Design review of the part built by this model. Coordinates are the model's own, in mm. A direction names the side the tool comes from. Give positions to 0.01 mm unless a question says otherwise; leave off trailing zeros. Loops run counter-clockwise (first coordinate to the right, second up) from the corner with the lowest first, then second, coordinate; pieces in that order, holes last. Notation, with made-up numbers: (14, 81.25) - (65, 81.25) arc R11 cw to (65, 86.25) - close; hole circle Ø6 at (42, 63). An arc over 180 degrees is marked (long way). Write each question's results on one line, items separated by ' | '.
Autodesk Inventor part; units mm, degrees
ref_plane "YZ Plane" through (0, 0, 0) normal (1, 0, 0) x (0, 1, 0)
ref_plane "XZ Plane" through (0, 0, 0) normal (0, 1, 0) x (-1, 0, 0)
ref_plane "XY Plane" through (0, 0, 0) normal (0, 0, 1) x (1, 0, 0)
sketch "Sketch1" plane through (0, 0, 0) normal (0, 1, 0) x (-1, 0, 0)
  circle A0 centre (0, 0) radius 10
  dimension "d0" = 20
extrude "Extrusion1" add sketch "Sketch1" along normal blind 2
sketch "Sketch2" plane through (0, 2, 0) normal (0, 1, 0) x (1, 0, 0)
  circle A0 centre (0, 0) radius 5.875
  dimension "d3" = 11.75
extrude "Extrusion2" cut sketch "Sketch2" against normal blind 1
sketch "Sketch3" plane through (0, 1, 0) normal (0, 1, 0) x (1, 0, 0)
  circle A0 centre (0, 0) radius 2
  dimension "d6" = 4
extrude "Extrusion3" cut sketch "Sketch3" against normal through all
properties part number "M3Bearing_Holder"
Item 1: We need section B-B on z = 0. Give the boundary of the cut face in (x, y) (3 decimals), then the cut area to 4 significant figures.
Output values:
outline: (-10, 0) - (-2, 0) - (-2, 1) - (-5.875, 1) - (-5.875, 2) - (-10, 2) - close; (2, 0) - (10, 0) - (10, 2) - (5.875, 2) - (5.875, 1) - (2, 1) - close | area: 24.25 mm²
Item 2: We need section D-D on x = 3. Give the boundary of the cut face in (y, z).
Output values:
outline: (0, -9.54) - (2, -9.54) - (2, -5.05) - (1, -5.05) - (1, 5.05) - (2, 5.05) - (2, 9.54) - (0, 9.54) - close
Item 3: Clearance check with flat-ended pins moving along their axes: P1, Ø3, axis at x = 0, z = 0, coming from the +Y side; P2, Ø3.5, axis at x = 0, z = 1, coming from the +Y side. State where each tip first meets the part, or that it passes through.
Output values:
P1: passes through | P2: stops at y = 1
Item 4: Draft analysis for pull direction X (two halves, no side actions). For faces 3 (the face through (2.17, 0.99, 9.76)), 4 (the face through (-0.434, 0.507, 1.952)), 5 (the face through (0.1, 0, 2.4)), state which applies: +X half, -X half, draft (parallel to the pull), parting line (faces both ways), or undercut.
Output values:
face 3: parting line | face 4: undercut | face 5: draft
Item 5: Tool access review of faces 1 (the face through (3, 1, 0)), 2 (the face through (-4.3, 2, -4.3)): name each direction out of +Z, -Z, +X, -X, +Y, -Y from which nothing blocks a thin tool from reaching the whole face with its end or side.
Output values:
face 1: +Y | face 2: +Z, -Z, +X, -X, +Y
Item 6: We need section A-A on x = 0. Give the boundary of the cut face in (y, z) (3 decimals).
Output values:
outline: (0, -10) - (2, -10) - (2, -5.875) - (1, -5.875) - (1, -2) - (0, -2) - close; (0, 2) - (1, 2) - (1, 5.875) - (2, 5.875) - (2, 10) - (0, 10) - close
Item 7: We need section C-C on y = 1.3. Give the boundary of the cut face in (x, z) (3 decimals), then the cut area to 3 significant figures.
Output values:
outline: circle Ø20 at (0, 0); hole circle Ø11.75 at (0, 0) | area: 206 mm²
Item 8: Wall thickness on probe 1 along Z at (x, y) = (0, 0.4); probe 2 along Y at (x, z) = (1.75, 5); probe 3 along Z at (x, y) = (0, 1.6) (3 decimals): over which ranges is each line inside the solid? List them lowest first.
Output values:
probe 1: z = -10 to -2, 2 to 10 | probe 2: y = 0 to 1 | probe 3: z = -10 to -5.875, 5.875 to 10
